Design review of the part built by this model. Coordinates are the model's own, in mm. Face numbers are marked on the shaded views. A direction names the side the tool comes from. Round coordinates to 2 decimals unless told otherwise and drop trailing zeros. Write each loop counter-clockwise with the first axis right and the second up, starting at its lowest first coordinate (ties: lowest second). Pieces come first, ordered by that corner, then holes.
from build123d import *

# Parameters (mm, degrees)
F1_DEPTH = 76.2
F2_R     = 12.7
F3_DEPTH = 50.8
F4_DEPTH = 50.8


with BuildPart() as f1:
    # F0 (on Front) → F1 (new body)
    with BuildSketch(Plane.XZ):
        Polygon((-15.125556, 12.843926), (-40.525556, 12.843926), (-40.525556, -12.556074), (86.474444, -12.556074), (86.474444, 12.843926), (35.674444, 12.843926), (35.674444, 1.494974), (-15.125556, 1.494974), align=None)
    extrude(amount=F1_DEPTH)

    # F2 (on Top) → F3 (cut)
    with BuildSketch(Plane.XY):
        with Locations((61.074444, -38.1)):
            Circle(F2_R)
    extrude(amount=F3_DEPTH, mode=Mode.SUBTRACT)

    # F2 (on Top) → F4 (cut)
    with BuildSketch(Plane.XY):
        with Locations((61.074444, -38.1)):
            Circle(F2_R)
    extrude(amount=-F4_DEPTH, mode=Mode.SUBTRACT)


solid = f1.part
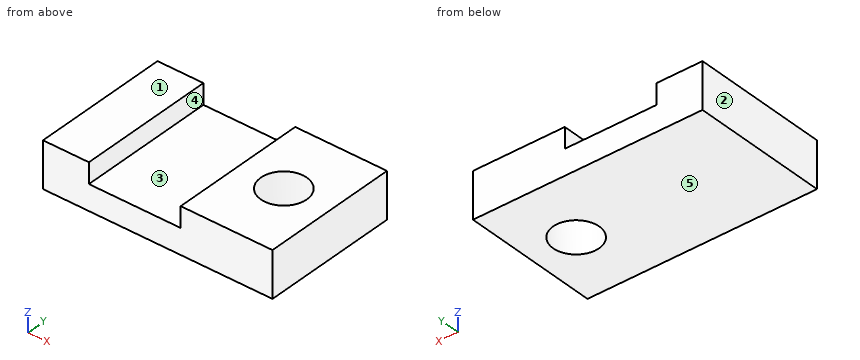
1) For line 1 along X through (y, z) = (-38.1, 5); line 2 along X through (y, z) = (-38.1, -1.75); line 3 along X through (y, z) = (-36.5, 9), list the stretches that pass through material, from the lowest coordinate up.
2) Add section C-C on y = -5. State the section outline as (x, z) points, and give its area (3 significant figures).
3) For the marked faces 4 and 5, list the 3-axis set-ups (+Z, -Z, +X, -X, +Y, -Y) from which the entire face can be reached by the end or side of a thin tool; tool diameter is ignored.
4) For P1, Ø1.5, axis at x = 26.5, y = -19.5, coming from the +Z side (3 decimals), flat-tipped, find the tip position at first contact; note if it passes through.
5) The part is to be moulded in two halves that separate along X. For the marked faces 1, 2 and 3, say which applies: pulls with the +X half, pulls with the -X half, needs draft (parallel to the pull), parting line crosses it, or undercut.
6) Add section A-A on z = 3.25. State the section outline as (x, y) points.
7) Add section D-D on z = -7.5. State the section outline as (x, y) points, and give its area (3 significant figures).
8) Add section B-B on y = -38.1. State the section outline as (x, z) points, and give its area (3 significant figures).
Computed:
1. line 1: x = -40.53 to -15.13, 35.67 to 48.37, 73.77 to 86.47
1. line 2: x = -40.53 to 48.37, 73.77 to 86.47
1. line 3: x = -40.53 to -15.13, 35.67 to 48.48, 73.67 to 86.47
2. outline: (-40.53, -12.56) - (86.47, -12.56) - (86.47, 12.84) - (35.67, 12.84) - (35.67, 1.49) - (-15.13, 1.49) - (-15.13, 12.84) - (-40.53, 12.84) - close
2. area: 2,650 mm2
3. face 4: +Z, +Y, -Y
3. face 5: -Z, +X, -X, +Y, -Y
4. P1: stops at z = 1.495
5. face 1: needs draft
5. face 2: pulls with the -X half
5. face 3: undercut
6. outline: (-40.53, -76.2) - (-15.13, -76.2) - (-15.13, 0) - (-40.53, 0) - close; (35.67, -76.2) - (86.47, -76.2) - (86.47, 0) - (35.67, 0) - close; hole circle Ø25.4 at (61.07, -38.1)
7. outline: (-40.53, -76.2) - (86.47, -76.2) - (86.47, 0) - (-40.53, 0) - close; hole circle Ø25.4 at (61.07, -38.1)
7. area: 9,170 mm2
8. outline: (-40.53, -12.56) - (48.37, -12.56) - (48.37, 12.84) - (35.67, 12.84) - (35.67, 1.49) - (-15.13, 1.49) - (-15.13, 12.84) - (-40.53, 12.84) - close; (73.77, -12.56) - (86.47, -12.56) - (86.47, 12.84) - (73.77, 12.84) - close
8. area: 2,000 mm2
